Geometry: final body of the model. Coordinates: model frame, mm. A direction names the side the tool comes from. Give positions to 0.01 mm unless a question says otherwise; leave off trailing zeros. Order: outer loops, then holes, each group sorted by start corner. A loop starts at its lowest first (then second) coordinate and runs counter-clockwise, first axis right, second up. Notation, with made-up numbers: (49, 0.5) - (57, 0.5) arc R21 ccw to (57, 22.5) - close; hole circle Ø4 at (21, 84). An arc over 180 degrees is marked (long way). One line per question, with ' | ' between items. Start each with the question number.
from build123d import *

# Parameters (mm, degrees)
SKETCH1_R               = 30
SKETCH1_R_2             = 25
BOSS_EXTRUDE1_DEPTH     = 180
SKETCH2_R               = 1.5
CUT_EXTRUDE1_DEPTH      = 31
CUT_EXTRUDE1_DEPTH_BACK = 31
SKETCH3_R               = 27
SKETCH3_R_2             = 19.569844271
CUT_EXTRUDE2_DEPTH      = 160


with BuildPart() as part:
    # Sketch1 → Boss-Extrude1 (new body)
    with BuildSketch(Plane(origin=(0, 0, 0), x_dir=(1, 0, 0), z_dir=(0, 1, 0))):
        Circle(SKETCH1_R)
        Circle(SKETCH1_R_2, mode=Mode.SUBTRACT)
    extrude(amount=BOSS_EXTRUDE1_DEPTH)

    # Sketch2 → Cut-Extrude1 (cut, two sides)
    with BuildSketch(Plane.XY) as cut_extrude1_sk:
        with Locations((0, 9.9)):
            Circle(SKETCH2_R)
    extrude(amount=CUT_EXTRUDE1_DEPTH, mode=Mode.SUBTRACT)
    extrude(cut_extrude1_sk.sketch, amount=-CUT_EXTRUDE1_DEPTH_BACK, mode=Mode.SUBTRACT)

    # Sketch3 → Cut-Extrude2 (cut)
    with BuildSketch(Plane(origin=(0, 180, 0), x_dir=(1, 0, 0), z_dir=(0, 1, 0))):
        Circle(SKETCH3_R)
        Circle(SKETCH3_R_2, mode=Mode.SUBTRACT)
    extrude(amount=-CUT_EXTRUDE2_DEPTH, mode=Mode.SUBTRACT)


solid = part.part
(1) Contact query for flat-ended pins moving along their axis: P1, Ø4, axis at x = -8.5, y = 136.5, coming from the -Z side; P2, Ø1, axis at x = -21.5, y = 132, coming from the -Z side; P3, Ø6, axis at x = 9, z = -18.5, coming from the +Y side; P4, Ø1.5, axis at x = -16, y = 61.5, coming from the +Z side. Output: stop coordinate, or through.
(2) Access query for faces 1 (the flat face through (-25, 180, -11)), 2 (the flat face through (24, 20, 8)). Directions: +Z, -Z, +X, -X, +Y, -Y. A direction counts if a zero-diameter tool reaches every point of the face in a straight line with its end or side. Return the directions, or none.
(3) Cut plane B-B, the plane x = 8.5. Return the cut outline in (y, z), plus the area to 3 significant figures.
(4) Pull-direction query (X, two-part tool) for faces 3 (the flat face through (-7, 0, -25)), 4 (the cylindrical face through (-29.97, 88.74, -1.32)), 5 (the cylindrical face through (-0.195, 11.387, -27.442)); classes: +X half, -X half, draft (parallel to the pull), parting line (faces both ways), or undercut.
(5) Material intervals for line 1 along Y through (x, z) = (0, -28.85); line 2 along X through (y, z) = (8.25, 0); line 3 along Z through (x, y) = (0, 144), sorted ascending. Write a range as from..to.
(6) Cut plane A-A, the plane z = 0. Return the cut outline in (x, y), plus the area to 3 significant figures.
(7) Cut plane C-C, the plane y = 165. Return the cut outline in (x, z), plus the area to 3 significant figures.
Results are:
1) P1: z = -29.29 | P2: z = -21.42 | P3: through | P4: z = 25.83
2) face 1: +Z, -Z, +X, -X, +Y | face 2: +Y
3) outline: (0, -28.77) - (180, -28.77) - (180, -25.63) - (20, -25.63) - (20, -23.51) - (0, -23.51) - close; (0, 23.51) - (20, 23.51) - (20, 25.63) - (180, 25.63) - (180, 28.77) - (0, 28.77) - close | area: 1,220 mm2
4) face 3: draft | face 4: parting line | face 5: undercut
5) line 1: 0..8.4, 11.4..180 | line 2: -30..-25, 25..30 | line 3: -30..-27, 27..30
6) outline: (-30, 0) - (-25, 0) - (-25, 20) - (-27, 20) - (-27, 180) - (-30, 180) - close; (25, 0) - (30, 0) - (30, 180) - (27, 180) - (27, 20) - (25, 20) - close | area: 1,160 mm2
7) outline: circle Ø60 at (0, 0); hole circle Ø54 at (0, 0) | area: 537 mm2
